from build123d import *

# Parameters (mm, degrees)
SALIENTE_EXTRUIR1_START   = -2.75
SALIENTE_EXTRUIR1_DEPTH   = 5.5
SALIENTE_EXTRUIR1_2_DEPTH = 2.75
SALIENTE_EXTRUIR2_DEPTH   = 38
SALIENTE_EXTRUIR3_START   = 2.75
SALIENTE_EXTRUIR3_DEPTH   = 2.75
CROQUIS4_W                = 23
CROQUIS4_H                = 43.5
CORTAR_EXTRUIR1_DEPTH     = 8.25
CORTAR_EXTRUIR2_DEPTH     = 2.75
CROQUIS6_W                = 38
CROQUIS6_H                = 22.249999999
CORTAR_EXTRUIR3_DEPTH     = 16.59246817
CROQUIS7_W                = 3.203765914
CROQUIS7_H                = 38
CORTAR_EXTRUIR4_DEPTH     = 8.25
CROQUIS8_W                = 3.203765916
CROQUIS8_H                = 38
CORTAR_EXTRUIR5_DEPTH     = 8.25
CROQUIS9_W                = 14
CROQUIS9_H                = 38
CORTAR_EXTRUIR6_DEPTH     = 0.703765915
CROQUIS10_W               = 14
CROQUIS10_H               = 38
CORTAR_EXTRUIR7_DEPTH     = 0.703765915
SALIENTE_EXTRUIR4_START   = 2.75
SALIENTE_EXTRUIR4_DEPTH   = 2.75
CORTAR_EXTRUIR8_DEPTH     = 2.75
CROQUIS13_W               = 12.249999999
CROQUIS13_H               = 2.75
CORTAR_EXTRUIR9_DEPTH     = 74.034358614
CROQUIS14_W               = 12.249999999
CROQUIS14_H               = 2.75
CORTAR_EXTRUIR10_DEPTH    = 74.034358614
CROQUIS15_W               = 5
CROQUIS15_H               = 2.75
CROQUIS16_W               = 5
CROQUIS16_H               = 2.75
TALADRO1_D                = 10.15
TALADRO1_DEPTH            = 2.75
TALADRO2_D                = 10.15


with BuildPart() as part:
    # Saliente-Extruir1: read off the stored shape, not the designer's step
    # Saliente-Extruir1 outline → Saliente-Extruir1 (new body)
    with BuildSketch(Plane(origin=(0, 40.75, 0), x_dir=(-1, 0, 0), z_dir=(0, 1, 0)).offset(SALIENTE_EXTRUIR1_START)):
        with BuildLine():
            Line((161.177139208, 19.345694485), (182.584423689, 27.755698719))
            Line((182.584423689, 27.755698719), (171.432026769, 56.143619441))
            ThreePointArc((171.432026769, 56.143619441), (156.523382412, 62.642259564), (150.024742289, 47.733615207))
            Line((150.024742289, 47.733615207), (161.177139208, 19.345694485))
        make_face()
    extrude(amount=SALIENTE_EXTRUIR1_DEPTH)

    # Saliente-Extruir1 2 outline → Saliente-Extruir1 2 (add)
    with BuildSketch(Plane(origin=(0, 40.75, 0), x_dir=(-1, 0, 0), z_dir=(0, 1, 0))):
        with BuildLine():
            ThreePointArc((161.177139208, 19.345694485), (176.085783565, 12.847054362), (182.584423687, 27.755698719))
            Line((182.584423687, 27.755698719), (161.177139208, 19.345694485))
        make_face()
    extrude(amount=SALIENTE_EXTRUIR1_2_DEPTH)

    # Croquis2 → Saliente-Extruir2 (add)
    with BuildSketch(Plane.XZ.offset(-38)):
        Polygon((-171.432026768, 56.143619442), (-150.024742288, 47.733615205), (-161.177139209, 19.345694483), (-182.584423689, 27.755698719), align=None)
    extrude(amount=SALIENTE_EXTRUIR2_DEPTH)

    # Croquis3 → Saliente-Extruir3 (add)
    with BuildSketch(Plane.XZ.offset(SALIENTE_EXTRUIR3_START)):
        with BuildLine():
            Line((-182.584423688, 27.755698719), (-171.432026768, 56.143619441))
            ThreePointArc((-171.432026768, 56.143619441), (-156.523382412, 62.642259564), (-150.024742289, 47.733615207))
            Line((-150.024742289, 47.733615207), (-161.177139208, 19.345694485))
            Line((-161.177139208, 19.345694485), (-182.584423688, 27.755698719))
        make_face()
    extrude(amount=-SALIENTE_EXTRUIR3_DEPTH)

    # Croquis4 → Cortar-Extruir1 (cut)
    with BuildSketch(Plane(origin=(-14.965700114, 0, -38.094511116), x_dir=(-0.9307514991056489, 0, 0.3656523580022251), z_dir=(-0.3656523580022251, 0, -0.9307514991056489))):
        with Locations((168.589662745, 19)):
            Rectangle(CROQUIS4_W, CROQUIS4_H)
    extrude(amount=-CORTAR_EXTRUIR1_DEPTH, mode=Mode.SUBTRACT)

    # Croquis5 → Cortar-Extruir2 (cut)
    with BuildSketch(Plane(origin=(0, 40.75, 0), x_dir=(1, 0, 0), z_dir=(0, 1, 0))):
        with BuildLine():
            Line((-161.142417183, -28.195858914), (-176.585881806, -34.262934025))
            ThreePointArc((-176.585881806, -34.262934025), (-167.602648859, -34.440489141), (-161.142417183, -28.195858914))
        make_face()
    extrude(amount=-CORTAR_EXTRUIR2_DEPTH, mode=Mode.SUBTRACT)

    # Croquis6 → Cortar-Extruir3 (cut)
    with BuildSketch(Plane(origin=(-149.193349022, 0, 58.611670162), x_dir=(0, 1, 0), z_dir=(0.9307514991056486, 0, -0.3656523580022258))):
        with Locations((19, -21.553766865)):
            Rectangle(CROQUIS6_W, CROQUIS6_H)
    extrude(amount=-CORTAR_EXTRUIR3_DEPTH, mode=Mode.SUBTRACT)

    # Croquis7 → Cortar-Extruir4 (cut)
    with BuildSketch(Plane(origin=(-3.8133032, 0, -9.706590403), x_dir=(0.9307514990825102, 0, -0.36565235806112356), z_dir=(0.36565235806112356, 0, 0.9307514990825102))):
        with Locations((-158.691545702, 19)):
            Rectangle(CROQUIS7_W, CROQUIS7_H)
    extrude(amount=-CORTAR_EXTRUIR4_DEPTH, mode=Mode.SUBTRACT)

    # Croquis8 → Cortar-Extruir5 (cut)
    with BuildSketch(Plane(origin=(-3.8133032, 0, -9.706590403), x_dir=(0.9307514990825102, 0, -0.36565235806112356), z_dir=(0.36565235806112356, 0, 0.9307514990825102))):
        with Locations((-178.487779787, 19)):
            Rectangle(CROQUIS8_W, CROQUIS8_H)
    extrude(amount=-CORTAR_EXTRUIR5_DEPTH, mode=Mode.SUBTRACT)

    # Croquis9 → Cortar-Extruir6 (cut)
    with BuildSketch(Plane(origin=(-164.636813645, 0, 64.678745273), x_dir=(-0.3656523580022247, 0, -0.930751499105649), z_dir=(0.930751499105649, 1.4355340193330324e-15, -0.3656523580022247))):
        with Locations((25.678766864, 19)):
            Rectangle(CROQUIS9_W, CROQUIS9_H)
    extrude(amount=-CORTAR_EXTRUIR6_DEPTH, mode=Mode.SUBTRACT)

    # Croquis10 → Cortar-Extruir7 (cut)
    with BuildSketch(Plane(origin=(-149.193349022, 0, 58.611670162), x_dir=(0.3656523580022248, 0, 0.930751499105649), z_dir=(-0.930751499105649, -1.4355340193330322e-15, 0.3656523580022248))):
        with Locations((-25.678766864, 19)):
            Rectangle(CROQUIS10_W, CROQUIS10_H)
    extrude(amount=-CORTAR_EXTRUIR7_DEPTH, mode=Mode.SUBTRACT)

    # Croquis11 → Saliente-Extruir4 (add)
    with BuildSketch(Plane.XZ.offset(2.75).offset(SALIENTE_EXTRUIR4_START)):
        with BuildLine():
            Line((-150.024742289, 47.733615207), (-161.177139208, 19.345694485))
            ThreePointArc((-161.177139208, 19.345694485), (-176.085783565, 12.847054362), (-182.584423687, 27.755698719))
            Line((-182.584423687, 27.755698719), (-171.432026769, 56.143619441))
            ThreePointArc((-171.432026769, 56.143619441), (-156.523382412, 62.642259564), (-150.024742289, 47.733615207))
        make_face()
    extrude(amount=-SALIENTE_EXTRUIR4_DEPTH)

    # Croquis12 → Cortar-Extruir8 (cut)
    with BuildSketch(Plane(origin=(0, 0, 0), x_dir=(-1, 0, 0), z_dir=(0, 1, 0))):
        with BuildLine():
            Line((161.142417183, 28.195858914), (176.585881806, 34.262934025))
            ThreePointArc((176.585881806, 34.262934025), (167.602648859, 34.440489141), (161.142417183, 28.195858914))
        make_face()
    extrude(amount=-CORTAR_EXTRUIR8_DEPTH, mode=Mode.SUBTRACT)

    # Croquis13 → Cortar-Extruir9 (cut, through all)
    with BuildSketch(Plane(origin=(-146.211439094, 0, 57.440205601), x_dir=(-0.36565235800222584, 0, -0.9307514991056486), z_dir=(0.9307514991056486, 0, -0.36565235800222584))):
        with Locations((16.553766864, -4.125)):
            Rectangle(CROQUIS13_W, CROQUIS13_H)
    extrude(amount=-CORTAR_EXTRUIR9_DEPTH, mode=Mode.SUBTRACT)

    # Croquis14 → Cortar-Extruir10 (cut, through all)
    with BuildSketch(Plane(origin=(-146.211439094, 0, 57.440205601), x_dir=(-0.36565235800222584, 0, -0.9307514991056486), z_dir=(0.9307514991056486, 0, -0.36565235800222584))):
        with Locations((16.553766864, 42.125)):
            Rectangle(CROQUIS14_W, CROQUIS14_H)
    extrude(amount=-CORTAR_EXTRUIR10_DEPTH, mode=Mode.SUBTRACT)

    # Croquis15 → Revolución1 (revolve)
    with BuildSketch(Plane(origin=(0, 0, 51.938617325), x_dir=(-1, 0, 0), z_dir=(0, 0, -1))):
        with Locations((158.228384529, -4.125)):
            Rectangle(CROQUIS15_W, CROQUIS15_H)
    revolve(axis=Axis((-160.728384529, -5.5, 51.938617325), (0, 1, 0)))

    # Croquis16 → Revolución2 (revolve)
    with BuildSketch(Plane(origin=(0, 0, 51.938617325), x_dir=(-1, 0, 0), z_dir=(0, 0, -1))):
        with Locations((158.228384529, 42.125)):
            Rectangle(CROQUIS16_W, CROQUIS16_H)
    revolve(axis=Axis((-160.728384529, 40.75, 51.938617325), (0, 1, 0)))

    # Taladro1
    with Locations(Plane(origin=(0, -5.5, 0), x_dir=(-1, 0, 0), z_dir=(0, -1, 0))):
        with Locations((171.880781448, -23.550696602)):
            Hole(TALADRO1_D / 2, depth=TALADRO1_DEPTH)

    # Taladro2 (through all)
    with Locations(Plane(origin=(0, 40.75, 0), x_dir=(-1, 0, 0), z_dir=(0, -1, 0))):
        with Locations((171.880781448, -23.550696602)):
            Hole(TALADRO2_D / 2)


solid = part.part
Could you check a few things on this model? Use its own coordinates, in mm. A direction names the side the tool comes from. Give positions to 0.01 mm unless a question says otherwise; leave off trailing zeros. Order: outer loops, then holes, each group sorted by start corner. A loop starts at its lowest first (then second) coordinate and runs counter-clockwise, first axis right, second up. Notation, with made-up numbers: (-8.75, -35.5) - (38.25, -35.5) arc R35 cw to (38.25, -2.5) - close; hole circle Ø11 at (-6, 16). An arc over 180 degrees is marked (long way). Return JSON: item names as keys, results as strings. Group by question number.
Q1. Please list where these lines run through material, in increasing order: line 1 along Y through (x, z) = (-179, 18); line 2 along Y through (x, z) = (-167, 61.5); line 3 along X through (y, z) = (30.5, 38). Write a range as [from, to].
Q2. Suppose I cut it at A-A, the plane y = 9.5. Please give me the cut outline in (x, z).
Q3. Suppose I cut it at B-B, the plane x = -151.5. Please give me the cut outline in (y, z).
Q4. Suppose I cut it at C-C, the plane z = 55. Please give me the cut outline in (x, y).
Q5. Which directions (+Z, -Z, +X, -X, +Y, -Y) give clear straight access to the entire face, cutting with the end or side of a thin tool? Please do faces 5 (the face through (-165.06, -4.14, 40.48)), 6 (the face through (-162.454, 42.144, 47.246)), 7 (the face through (-173.302, 19.266, 48.014)), 8 (the face through (-165.06, 42.11, 40.48)).
Q6. Thinking about a two-plate mould opening in Z: for faces 1 (the face through (-174.646, 19.266, 41.127)), 2 (the face through (-163, -2.75, 46)), 3 (the face through (-175.849, 42.106, 12.757)), 4 (the face through (-168.365, -4.144, 54.939)), which applies, pulls with the +Z half, pulls with the -Z half, needs draft (parallel to the pull), parting line crosses it, or undercut?
Q7. Will these pins go through, and if not, where does the flat tip stop? pin 1 Ø12 at (y, z) = (28.5, 43.5) entering from -X; pin 2 Ø11.5 at (x, z) = (-171.5, 23) entering from -Y; pin 3 Ø3 at (y, z) = (0, 27) entering from -X; pin 4 Ø12 at (x, y) = (-179.5, 24.5) entering from +Z.
Q8. Suppose I cut it at D-D, the plane x = -168. Please give me the cut outline in (y, z).
Resolved:
{
 "1": {"line 1": "y = [-5.5, -2.75], [40.75, 43.5]", "line 2": "y = [-5.5, 0], [38, 43.5]", "line 3": "x = [-178.56, -175.87], [-156.53, -153.85]"},
 "2": {"outline": "(-179.57, 35.43) - (-177.24, 34.52) - (-172.12, 47.55) - (-174.45, 48.46) - close; (-160.49, 27.94) - (-158.16, 27.02) - (-153.04, 40.05) - (-155.37, 40.97) - close"},
 "3": {"outline": "(-5.5, 48.31) - (-2.75, 48.31) - (-2.75, 43.98) - (0, 43.98) - (0, 58.8) - (-5.5, 58.8) - close; (38, 43.98) - (40.75, 43.98) - (40.75, 48.31) - (43.5, 48.31) - (43.5, 58.8) - (38, 58.8) - close"},
 "4": {"outline": "(-171.88, -2.75) - (-168.52, -2.75) - (-168.52, -5.5) - (-149.64, -5.5) - (-149.64, 0) - (-171.88, 0) - close; (-171.88, 38) - (-149.64, 38) - (-149.64, 43.5) - (-168.52, 43.5) - (-168.52, 40.75) - (-171.88, 40.75) - close"},
 "5": {"face 5": "+X, -Y", "face 6": "+Y", "face 7": "+Z, +X", "face 8": "+X, +Y"},
 "6": {"face 1": "pulls with the -Z half", "face 2": "undercut", "face 3": "parting line crosses it", "face 4": "undercut"},
 "7": {"pin 1": "stops at x = -178.76", "pin 2": "stops at y = -5.5", "pin 3": "stops at x = -161.28", "pin 4": "stops at z = 48.46"},
 "8": {"outline": "(-5.5, 12.73) - (-2.75, 12.73) - (-2.75, 20.28) - (-5.5, 20.28) - close; (-5.5, 26.82) - (-2.75, 26.82) - (-2.75, 34.59) - (0, 34.59) - (0, 60.85) - (-5.5, 60.85) - (-5.5, 54.8) - (-2.75, 54.8) - (-2.75, 41.63) - (-5.5, 41.63) - close; (38, 34.59) - (40.75, 34.59) - (40.75, 26.82) - (43.5, 26.82) - (43.5, 41.63) - (40.75, 41.63) - (40.75, 54.8) - (43.5, 54.8) - (43.5, 60.85) - (38, 60.85) - close; (40.75, 12.73) - (43.5, 12.73) - (43.5, 20.28) - (40.75, 20.28) - close"}
}
